```python
from build123d import *

# Parameters (mm, degrees)
MODEL_W             = 232.41
MODEL_H             = 163.2712
MODEL_R             = 2.766686572
MODEL_R_2           = 5.865375533
BOSS_EXTRUDE2_DEPTH = 1.5748
SKETCH10_W          = 76.2
SKETCH10_H          = 25.4
CUT_EXTRUDE13_DEPTH = 1.5748
SKETCH11_R          = 1.2446
CUT_EXTRUDE14_DEPTH = 279.870205617


with BuildPart() as part:
    # Model → Boss-Extrude2 (new body)
    with BuildSketch(Plane.XY):
        with Locations((80.00320848, 116.527086979)):
            Rectangle(MODEL_W, MODEL_H)
        with Locations((-4.104063311, 147.485885883)):
            Circle(MODEL_R, mode=Mode.SUBTRACT)
        with Locations((68.936462192, 92.041486979)):
            Circle(MODEL_R_2, mode=Mode.SUBTRACT)
        with Locations((2.535984462, 92.041486979)):
            Circle(MODEL_R_2, mode=Mode.SUBTRACT)
        with Locations((24.669477039, 92.041486979)):
            Circle(MODEL_R_2, mode=Mode.SUBTRACT)
        with Locations((46.802969616, 92.041486979)):
            Circle(MODEL_R_2, mode=Mode.SUBTRACT)
        with Locations((91.069954769, 92.041486979)):
            Circle(MODEL_R_2, mode=Mode.SUBTRACT)
        with Locations((113.203447345, 92.041486979)):
            Circle(MODEL_R_2, mode=Mode.SUBTRACT)
        with Locations((135.336939922, 92.041486979)):
            Circle(MODEL_R_2, mode=Mode.SUBTRACT)
        with Locations((157.470432499, 92.041486979)):
            Circle(MODEL_R_2, mode=Mode.SUBTRACT)
        with Locations((146.40368621, 114.174979556)):
            Circle(MODEL_R_2, mode=Mode.SUBTRACT)
        with Locations((124.270193634, 114.174979556)):
            Circle(MODEL_R_2, mode=Mode.SUBTRACT)
        with Locations((102.136701057, 114.174979556)):
            Circle(MODEL_R_2, mode=Mode.SUBTRACT)
        with Locations((80.00320848, 114.174979556)):
            Circle(MODEL_R_2, mode=Mode.SUBTRACT)
        with Locations((57.869715904, 114.174979556)):
            Circle(MODEL_R_2, mode=Mode.SUBTRACT)
        with Locations((35.736223327, 114.174979556)):
            Circle(MODEL_R_2, mode=Mode.SUBTRACT)
        with Locations((13.602730751, 114.174979556)):
            Circle(MODEL_R_2, mode=Mode.SUBTRACT)
        with BuildLine():
            Line((28.016503786, 169.309509564), (38.374978312, 169.309509564))
            ThreePointArc((38.374978312, 169.309509564), (38.406279807, 169.296544074), (38.419245297, 169.265242579))
            Line((38.419245297, 169.265242579), (38.419245297, 158.906768053))
            ThreePointArc((38.419245297, 158.906768053), (38.406279807, 158.875466558), (38.374978312, 158.862501068))
            Line((38.374978312, 158.862501068), (28.016503786, 158.862501068))
            ThreePointArc((28.016503786, 158.862501068), (27.985202291, 158.875466558), (27.972236801, 158.906768053))
            Line((27.972236801, 158.906768053), (27.972236801, 169.265242579))
            ThreePointArc((27.972236801, 169.265242579), (27.985202291, 169.296544074), (28.016503786, 169.309509564))
        make_face(mode=Mode.SUBTRACT)
        with BuildLine():
            Line((28.016503786, 136.109270699), (38.374978312, 136.109270699))
            ThreePointArc((38.374978312, 136.109270699), (38.406279807, 136.096305209), (38.419245297, 136.065003714))
            Line((38.419245297, 136.065003714), (38.419245297, 125.706529188))
            ThreePointArc((38.419245297, 125.706529188), (38.406279807, 125.675227693), (38.374978312, 125.662262203))
            Line((38.374978312, 125.662262203), (28.016503786, 125.662262203))
            ThreePointArc((28.016503786, 125.662262203), (27.985202291, 125.675227693), (27.972236801, 125.706529188))
            Line((27.972236801, 125.706529188), (27.972236801, 136.065003714))
            ThreePointArc((27.972236801, 136.065003714), (27.985202291, 136.096305209), (28.016503786, 136.109270699))
        make_face(mode=Mode.SUBTRACT)
        with BuildLine():
            Line((44.616623219, 152.709390132), (54.975097745, 152.709390132))
            ThreePointArc((54.975097745, 152.709390132), (55.00639924, 152.696424641), (55.01936473, 152.665123146))
            Line((55.01936473, 152.665123146), (55.01936473, 142.306648621))
            ThreePointArc((55.01936473, 142.306648621), (55.00639924, 142.275347125), (54.975097745, 142.262381635))
            Line((54.975097745, 142.262381635), (44.616623219, 142.262381635))
            ThreePointArc((44.616623219, 142.262381635), (44.585321724, 142.275347125), (44.572356234, 142.306648621))
            Line((44.572356234, 142.306648621), (44.572356234, 152.665123146))
            ThreePointArc((44.572356234, 152.665123146), (44.585321724, 152.696424641), (44.616623219, 152.709390132))
        make_face(mode=Mode.SUBTRACT)
        with BuildLine():
            Line((21.819125865, 152.665123146), (21.819125865, 142.306648621))
            ThreePointArc((21.819125865, 142.306648621), (21.806160375, 142.275347125), (21.77485888, 142.262381635))
            Line((21.77485888, 142.262381635), (11.416384354, 142.262381635))
            ThreePointArc((11.416384354, 142.262381635), (11.385082859, 142.275347125), (11.372117369, 142.306648621))
            Line((11.372117369, 142.306648621), (11.372117369, 152.665123146))
            ThreePointArc((11.372117369, 152.665123146), (11.385082859, 152.696424641), (11.416384354, 152.709390132))
            Line((11.416384354, 152.709390132), (21.77485888, 152.709390132))
            ThreePointArc((21.77485888, 152.709390132), (21.806160375, 152.696424641), (21.819125865, 152.665123146))
        make_face(mode=Mode.SUBTRACT)
        with BuildLine():
            Line((146.071683822, 154.070599925), (146.071683822, 141.963579486))
            ThreePointArc((146.071683822, 141.963579486), (146.058718332, 141.93227799), (146.027416836, 141.9193125))
            Line((146.027416836, 141.9193125), (90.339549514, 141.9193125))
            ThreePointArc((90.339549514, 141.9193125), (90.308248019, 141.93227799), (90.295282529, 141.963579486))
            Line((90.295282529, 141.963579486), (90.295282529, 154.070599925))
            ThreePointArc((90.295282529, 154.070599925), (90.308248019, 154.10190142), (90.339549514, 154.11486691))
            Line((90.339549514, 154.11486691), (146.027416836, 154.11486691))
            ThreePointArc((146.027416836, 154.11486691), (146.058718332, 154.10190142), (146.071683822, 154.070599925))
        make_face(mode=Mode.SUBTRACT)
    extrude(amount=BOSS_EXTRUDE2_DEPTH)

    # Sketch10 → Cut-Extrude13 (cut)
    with BuildSketch(Plane.XY.offset(1.5748)):
        with Locations((118.183483175, 148.017089705)):
            Rectangle(SKETCH10_W, SKETCH10_H)
    extrude(amount=-CUT_EXTRUDE13_DEPTH, mode=Mode.SUBTRACT)

    # Sketch11 → Cut-Extrude14 (cut, through all)
    with BuildSketch(Plane(origin=(0, 0, 0), x_dir=(-1, 0, 0), z_dir=(0, 0, -1))):
        with Locations((-155.610383175, 163.523789705)):
            Circle(SKETCH11_R)
        with Locations((-155.610383175, 132.510389705)):
            Circle(SKETCH11_R)
        with Locations((-80.578783175, 132.510389705)):
            Circle(SKETCH11_R)
        with Locations((-80.578783175, 163.523789705)):
            Circle(SKETCH11_R)
    extrude(amount=-CUT_EXTRUDE14_DEPTH, mode=Mode.SUBTRACT)


solid = part.part
```
Work out the finished part from the listing and answer in its coordinate system (mm). Round coordinates to 2 decimals unless told otherwise and drop trailing zeros. Order: outer loops, then holes, each group sorted by start corner. A loop starts at its lowest first (then second) coordinate and runs counter-clockwise, first axis right, second up.
Q1. A cutting plane is placed at A-A, the plane x = 14.5. Determine the outline of the cut face in (y, z), then the cut area to 3 significant figures.
Solution:
outline: (34.89, 0) - (108.38, 0) - (108.38, 1.57) - (34.89, 1.57) - close; (119.97, 0) - (142.26, 0) - (142.26, 1.57) - (119.97, 1.57) - close; (152.71, 0) - (198.16, 0) - (198.16, 1.57) - (152.71, 1.57) - close
area: 222 mm2
Q2. Given pin 1 Ø10.5 at (x, y) = (24.67, 92.04) entering from -Z, flat-ended and moving along its own axis, determine where the tip first touches the part or whether it passes through.
Solution:
pin 1: passes through
Q3. Find the intervals of material crossed by line 1 along Y through (x, z) = (91.5, 0.95); line 2 along Y through (x, z) = (84, 0.8); line 3 along X through (y, z) = (145.5, 1.2), in increasing order.
Solution:
line 1: y = 34.89 to 86.19, 97.89 to 135.32, 160.72 to 198.16
line 2: y = 34.89 to 109.88, 118.47 to 135.32, 160.72 to 198.16
line 3: x = -36.2 to -6.03, -2.18 to 11.37, 21.82 to 44.57, 55.02 to 80.08, 156.28 to 196.21
Q4. A cutting plane is placed at C-C, the plane x = 102. Determine the outline of the cut face in (y, z).
Solution:
outline: (34.89, 0) - (108.31, 0) - (108.31, 1.57) - (34.89, 1.57) - close; (120.04, 0) - (135.32, 0) - (135.32, 1.57) - (120.04, 1.57) - close; (160.72, 0) - (198.16, 0) - (198.16, 1.57) - (160.72, 1.57) - close
Q5. A cutting plane is placed at B-B, the plane y = 117. Count the separate pieces of the cut face and the enclosed holes in it, then the cut area to 3 significant figures.
Solution:
separate pieces: 8
enclosed holes: 0
area: 253 mm2
Q6. The mould has two halves that part along Y. Classify faces 1 (the flat face through (78, 100, 1.575)), 2 (the cylindrical face through (9.28, 118.14, 0.78)): pulls with the +Y half, pulls with the -Y half, needs draft (parallel to the pull), parting line crosses it, or undercut.
Solution:
face 1: needs draft
face 2: undercut
